from build123d import *

# Parameters (mm, degrees)
HEX_CUT_DEPTH = 1.25


with BuildPart() as part:
    # Body_Sketch → Body_Revolve (revolve)
    with BuildSketch(Plane(origin=(0, 0, 0), x_dir=(0, 0, -1), z_dir=(1, 0, 0)), mode=Mode.PRIVATE) as body_revolve_sk:
        with BuildLine():
            Line((8, 0), (8, 1))
            Line((8, 1), (7.75, 1.25))
            Line((7.75, 1.25), (0.1, 1.25))
            ThreePointArc((0.1, 1.25), (0.029289322, 1.279289322), (0, 1.35))
            Line((0, 1.35), (0, 2.25))
            Line((0, 2.25), (-2.25, 2.25))
            Line((-2.25, 2.25), (-2.5, 1.816987298))
            Line((-2.5, 1.816987298), (-2.5, 0))
            Line((-2.5, 0), (8, 0))
        make_face()
    revolve(body_revolve_sk.sketch.rotate(Axis((0, 0, 0), (0, 0, -1)), 90), axis=Axis((0, 0, 0), (0, 0, -1)))

    # Key_Sketch → Hex_Cut (cut)
    with BuildSketch(Plane.XY.offset(2.5)):
        Polygon((1.154700538, 0), (0.577350269, 1), (-0.577350269, 1), (-1.154700538, 0), (-0.577350269, -1), (0.577350269, -1), align=None)
    extrude(amount=-HEX_CUT_DEPTH, mode=Mode.SUBTRACT)


solid = part.part
Read the model definition and answer for the solid it produces. Units are mm, in the model's axes. A direction names the side the tool comes from. Give positions to 0.01 mm unless a question says otherwise; leave off trailing zeros. Write each loop counter-clockwise with the first axis right and the second up, starting at its lowest first coordinate (ties: lowest second). Pieces come first, ordered by that corner, then holes. Notation, with made-up numbers: (-3, -19.5) - (11, -19.5) arc R32 ccw to (11, 10.5) - close; hole circle Ø7 at (-4.5, -12). An arc over 180 degrees is marked (long way). Answer in a Markdown table with one row per item. Add a question column.
Item 1: A flat-ended cylindrical pin translates along its axis: P1, Ø0.6, axis at x = -0.5, y = 0, coming from the +Z side. Find the tip coordinate at first contact, or state that the pin passes through.
Item 2: Determine the mould class of faces 4 (the face through (0, 0, 1.25)), 5 (the face through (0, 0, -8)), 6 (the face through (-1.66, -1.52, 1.14)), 7 (the face through (-0.86, 0.51, 1.88)) for opening direction X: pulls with the +X half, pulls with the -X half, needs draft (parallel to the pull), parting line crosses it, or undercut.
Item 3: Find the intervals of material crossed by L1, parallel to Z at x = 0.55, y = -0.1; L2, parallel to Z at x = 0, y = 1.8; L3, parallel to Y at x = 0.45, z = 1.5, in increasing order.
Item 4: Section A-A, the plane x = 0 is taken. Write down the section's boundary in (y, z), and give its area (3 significant figures).
Item 5: Section B-B, the plane z = -4.25 is taken. Write down the section's boundary in (x, y), and give its area (3 significant figures).
Item 6: A tool of negligible diameter and unlimited length cuts with its end or side. For faces 1 (the face through (1, 1, 2.5)), 2 (the face through (-0.5, 1.5, 0)), 3 (the face through (0.86, -0.51, 1.88)), from which of +Z, -Z, +X, -X, +Y, -Y can it reach the whole face along a straight path? Write none if from no direction.
Recorded:
| question | item | result |
|---|---|---|
| 1 | P1 | stops at z = 1.25 |
| 2 | face 4 | undercut |
| 2 | face 5 | needs draft |
| 2 | face 6 | parting line crosses it |
| 2 | face 7 | undercut |
| 3 | L1 | z = -8 to 1.25 |
| 3 | L2 | z = 0 to 2.5 |
| 3 | L3 | y = -2.2 to -1, 1 to 2.2 |
| 4 | outline | (-2.25, 0) - (-1.35, 0) arc R0.1 cw to (-1.25, -0.1) - (-1.25, -7.75) - (-1, -8) - (1, -8) - (1.25, -7.75) - (1.25, -0.1) arc R0.1 cw to (1.35, 0) - (2.25, 0) - (2.25, 2.25) - (1.82, 2.5) - (1, 2.5) - (1, 1.25) - (-1, 1.25) - (-1, 2.5) - (-1.82, 2.5) - (-2.25, 2.25) - close |
| 4 | area | 28.6 mm2 |
| 5 | outline | circle Ø2.5 at (0, 0) |
| 5 | area | 4.91 mm2 |
| 6 | face 1 | +Z, +X, -X, +Y, -Y |
| 6 | face 2 | -Z |
| 6 | face 3 | +Z |
